Could you check a few things on this model? Use its own coordinates, in mm. Face numbers are marked on the shaded views. A direction names the side the tool comes from. Give positions to 0.01 mm unless a question says otherwise; leave off trailing zeros. Loops run counter-clockwise (first coordinate to the right, second up) from the corner with the lowest first, then second, coordinate; pieces in that order, holes last. Notation, with made-up numbers: M 11,38.5 L 41,38.5 A16 cw 41,65.5 Z; hole C -10,-17.5 d4. An arc over 180 degrees is marked long. Use CSV: the item, a comma, the result in double quotes.
```python
from build123d import *

# Parameters (mm, degrees)
F3_DEPTH = 2.4


with BuildPart() as f1:
    # F0 (on Front) → F1 (revolve)
    with BuildSketch(Plane.XZ):
        Polygon((-130.5134040415, -110.4772146098), (-130.5134040415, -122.0772146098), (-119.5134040415, -122.0772146098), (-119.5134040415, -94.0772146098), (-122.9134040415, -94.0772146098), (-122.9134040415, -103.0772146098), (-130.5134040415, -103.0772146098), (-130.5134040415, -108.0772146098), (-141.5134040415, -108.0772146098), (-141.5134040415, -110.4772146098), align=None)
    revolve(axis=Axis((-119.5134040415, 0, -108.0772146098), (0, 0, -1)))

    # F2 (on face) → F3 (cut, through all)
    with BuildSketch(Plane.XY.offset(-108.0772146098)):
        with BuildLine():
            ThreePointArc((-121.0167680789, 16.9876935094), (-121.0259896486, 17.2106541317), (-121.0535913671, 17.4320917564))
            ThreePointArc((-121.0535913671, 17.4320917564), (-123.7167680789, 16.9876935094), (-126.27988757, 16.1389188194))
            ThreePointArc((-126.27988757, 16.1389188194), (-123.2868975321, 14.3221332844), (-121.0167680789, 16.9876935094))
        make_face()
        with BuildLine():
            ThreePointArc((-126.27988757, 16.1389188194), (-123.7167680789, 16.9876935094), (-121.0535913671, 17.4320917564))
            ThreePointArc((-121.0535913671, 17.4320917564), (-124.3652871018, 19.6086519366), (-126.27988757, 16.1389188194))
        make_face()
        with BuildLine():
            ThreePointArc((-99.8403964321, -4.2622778759), (-100.4770477105, -2.5208439688), (-102.0867609158, -1.6006590418))
            ThreePointArc((-102.0867609158, -1.6006590418), (-102.5403964321, -4.2622778759), (-103.3980588072, -6.8224370996))
            ThreePointArc((-103.3980588072, -6.8224370996), (-100.9633245271, -6.4538171082), (-99.8403964321, -4.2622778759))
        make_face()
        with BuildLine():
            ThreePointArc((-103.3980588072, -6.8224370996), (-102.5403964321, -4.2622778759), (-102.0867609158, -1.6006590418))
            ThreePointArc((-102.0867609158, -1.6006590418), (-105.1590890347, -3.6046692894), (-103.3980588072, -6.8224370996))
        make_face()
        with BuildLine():
            ThreePointArc((-129.8403964321, -11.6853527655), (-131.3455427368, -9.2641289744), (-134.1828591335, -9.5423837329))
            ThreePointArc((-134.1828591335, -9.5423837329), (-132.5403964321, -11.6853527655), (-130.5878381405, -13.550162707))
            ThreePointArc((-130.5878381405, -13.550162707), (-130.0342133395, -12.6898657352), (-129.8403964321, -11.6853527655))
        make_face()
        with BuildLine():
            ThreePointArc((-130.5878381405, -13.550162707), (-132.5403964321, -11.6853527655), (-134.1828591335, -9.5423837329))
            ThreePointArc((-134.1828591335, -9.5423837329), (-134.5502752581, -13.4882357636), (-130.5878381405, -13.550162707))
        make_face()
    extrude(amount=-F3_DEPTH, mode=Mode.SUBTRACT)


solid = f1.part
```
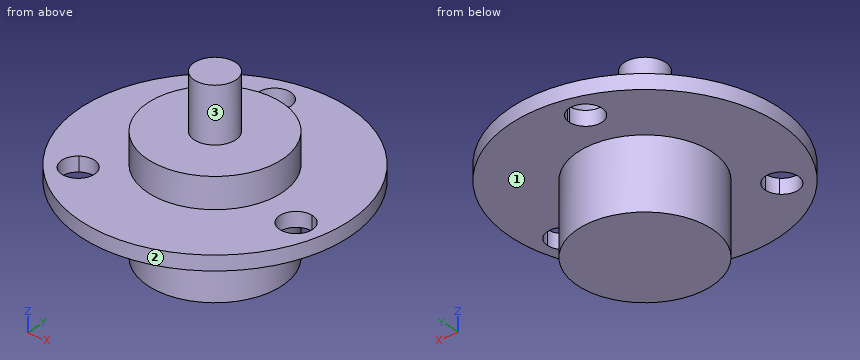
1. I want a section at C-C, the plane y = 0. List the corners of the cut face in (x, z) for me.
Outcome:
outline,"M -141.51,-110.48 L -130.51,-110.48 L -130.51,-122.08 L -108.51,-122.08 L -108.51,-110.48 L -97.51,-110.48 L -97.51,-108.08 L -108.51,-108.08 L -108.51,-103.08 L -116.11,-103.08 L -116.11,-94.08 L -122.91,-94.08 L -122.91,-103.08 L -130.51,-103.08 L -130.51,-108.08 L -141.51,-108.08 Z"
2. Which directions (+Z, -Z, +X, -X, +Y, -Y) give clear straight access to the entire face, cutting with the end or side of a thin tool? Please do the marked faces 1, 2 and 3.
Outcome:
face 1,"-Z"
face 2,"+Z, -Z"
face 3,"+Z"
3. Please list where these lines run through material, in increasing order: line 1 (Z direction, x = -128.5, y = -18.5); line 2 (Y direction, x = -134, z = -108.5); line 3 (Y direction, x = -122.5, z = -103.25).
Outcome:
line 1,"-110.48 to -108.08"
line 2,"-16.56 to -13.96, -9.41 to 16.56"
line 3,"-10.59 to 10.59"
4. I'm going to push flat-ended pins straight in: pin 1 Ø8 at (y, z) = (-9, -110.5) entering from +X; pin 2 Ø6 at (y, z) = (13, -117) entering from -X; pin 3 Ø8 at (x, y) = (-129, 16.5) entering from -Z. Where does each tip first touch, or does it pass through?
Outcome:
pin 1,"x = -98.09"
pin 2,"x = -124.1"
pin 3,"z = -110.48"
5. I want a section at D-D, the plane z = -97. List the corners of the cut face in (x, y) for me.
Outcome:
outline,"C -119.51,0 d6.8"
6. I want a section at A-A, the plane y = -12.5. List the corners of the cut face in (x, z) for me, then the cut area to 3 significant figures.
Outcome:
outline,"M -137.62,-110.48 L -135.11,-110.48 L -135.11,-108.08 L -137.62,-108.08 Z; M -129.97,-110.48 L -101.41,-110.48 L -101.41,-108.08 L -129.97,-108.08 Z"
area,"74.5 mm2"
7. I want a section at B-B, the plane x = -104.5. List the corners of the cut face in (y, z) for me.
Outcome:
outline,"M -16.08,-110.48 L -6.12,-110.48 L -6.12,-108.08 L -16.08,-108.08 Z; M -2.4,-110.48 L 16.08,-110.48 L 16.08,-108.08 L -2.4,-108.08 Z"
